Read the model definition and answer for the solid it produces. Units are mm, in the model's axes. Face numbers are marked on the shaded views. Give positions to 0.01 mm unless a question says otherwise; leave off trailing zeros. Order: outer loops, then holes, each group sorted by start corner. A loop starts at its lowest first (then second) coordinate and runs counter-clockwise, first axis right, second up. Notation, with made-up numbers: M 50,-20.5 L 105,-20.5 A25 ccw 105,17.5 Z; hole C 24.5,26.5 d10. An arc over 180 degrees is marked long. One line per item, written item: value.
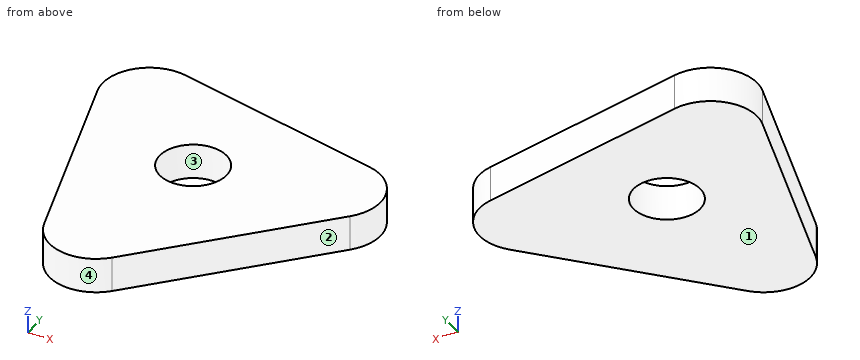
from build123d import *

# Parameters (mm, degrees)
F1_DEPTH = 7.62
F2_R     = 7.270124
F3_DEPTH = 25.4


with BuildPart() as f1:
    # F0 (on Top) → F1 (new body)
    with BuildSketch(Plane.XY):
        with BuildLine():
            ThreePointArc((-19.422231, 41.032927), (-29.168799, 38.16413), (-31.557632, 28.288955))
            Line((-31.557632, 28.288955), (-18.116118, -17.377788))
            ThreePointArc((-18.116118, -17.377788), (-10.758383, -24.384165), (-1.011814, -21.515368))
            Line((-1.011814, -21.515368), (31.815989, 12.958696))
            ThreePointArc((31.815989, 12.958696), (34.204821, 22.833871), (26.847086, 29.840248))
            Line((26.847086, 29.840248), (-19.422231, 41.032927))
        make_face()
    extrude(amount=F1_DEPTH)

    # F2 (on face) → F3 (cut)
    with BuildSketch(Plane.XY.offset(7.62)):
        with Locations((-2.968387, 14.133593)):
            Circle(F2_R)
    extrude(amount=-F3_DEPTH, mode=Mode.SUBTRACT)


solid = f1.part
1) Find section D-D, the plane x = 14. Write down the section's boundary in (y, z).
Reported:
outline: M -5.75,0 L 32.95,0 L 32.95,7.62 L -5.75,7.62 Z
2) Consider probe 1 along Y at (x, z) = (-3.5, 1); probe 2 along X at (y, z) = (8, 4.75); probe 3 along X at (y, z) = (-9.5, 1.25). Determine where each line is inside the solid, lowest interval first.
Reported:
probe 1: y = -23.43 to 6.88, 21.38 to 37.18
probe 2: x = -25.59 to -6.87, 0.93 to 27.09
probe 3: x = -20.43 to 10.43
3) Determine the mould class of the marked faces 1, 2, 3 and 4 for opening direction X: +X half, -X half, draft (parallel to the pull), parting line (faces both ways), or undercut.
Reported:
face 1: draft
face 2: +X half
face 3: undercut
face 4: parting line
4) Find section C-C, the plane y = 17.5. Write down the section's boundary in (x, z), plus the area to 3 significant figures.
Reported:
outline: M -28.38,0 L -9.41,0 L -9.41,7.62 L -28.38,7.62 Z; M 3.48,0 L 34.31,0 L 34.31,7.62 L 3.48,7.62 Z
area: 380 mm^2
5) Each of these flat-tipped pins is pushed along its axis until it touches: pin 1 Ø10 at (x, y) = (5, 28) entering from -Z; pin 2 Ø1 at (y, z) = (18.5, 6.5) entering from +X; pin 3 Ø1 at (y, z) = (34.5, 6) entering from -X. Where does it stop, or does it pass through?
Reported:
pin 1: stops at z = 0
pin 2: stops at x = 34.57
pin 3: stops at x = -31.57
6) Find section A-A, the plane x = -2. Write down the section's boundary in (y, z), plus the area to 3 significant figures.
Reported:
outline: M -22.42,0 L 6.93,0 L 6.93,7.62 L -22.42,7.62 Z; M 21.34,0 L 36.82,0 L 36.82,7.62 L 21.34,7.62 Z
area: 342 mm^2
7) Find section B-B, the plane z = 2.25. Write down the section's boundary in (x, y).
Reported:
outline: M -31.56,28.29 L -18.12,-17.38 A10.16 ccw -1.01,-21.52 L 31.82,12.96 A10.16 ccw 26.85,29.84 L -19.42,41.03 A10.16 ccw Z; hole C -2.97,14.13 d14.54
